For this review, use the dimensioned drawing (mm, ordinates from the lowest corner) and the shaded views. A direction names the side the tool comes from. Coordinates: 2 decimals unless noted, no trailing zeros. Order: outer loops, then holes, each group sorted by start corner. A loop starts at its lowest first (then second) coordinate and runs counter-clockwise, first axis right, second up. Notation, with made-up numbers: M -23,55 L 3,55 A19 ccw 3,74 Z; hole C 32,50.25 d2. An arc over 180 degrees is marked long. Answer in a Markdown table with one row per item.
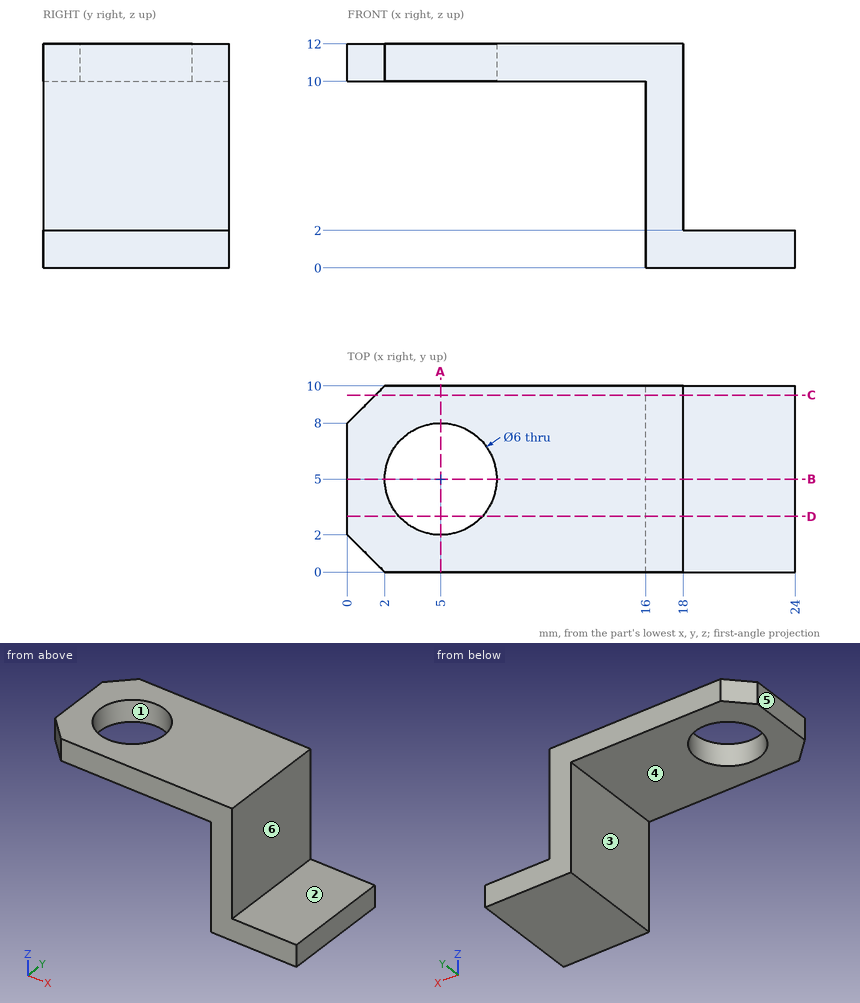
(1) Add section B-B, the plane y = 5. Give the boundary of the cut face in (x, z), and give its area (3 significant figures).
Return value:
| item | result |
|---|---|
| outline | M 0,10 L 2,10 L 2,12 L 0,12 Z; M 8,10 L 16,10 L 16,0 L 24,0 L 24,2 L 18,2 L 18,12 L 8,12 Z |
| area | 56.0 mm2 |
(2) Insertion check: pin 1 Ø5 at (y, z) = (4.5, 3) entering from -X; pin 2 Ø1.8 at (x, y) = (21, 4.5) entering from +Z; pin 3 Ø5 at (y, z) = (4, 7.5) entering from +X. Each pin has a flat end and moves straight along its axis. Give the tip position at first contact, or say it passes through.
Return value:
| item | result |
|---|---|
| pin 1 | stops at x = 16 |
| pin 2 | stops at z = 2 |
| pin 3 | stops at x = 18 |
(3) Add section D-D, the plane y = 3. Give the boundary of the cut face in (x, z).
Return value:
| item | result |
|---|---|
| outline | M 0,10 L 2.76,10 L 2.76,12 L 0,12 Z; M 7.24,10 L 16,10 L 16,0 L 24,0 L 24,2 L 18,2 L 18,12 L 7.24,12 Z |
(4) Draft analysis for pull direction X (two halves, no side actions). For the marked faces 1, 2 and 3, state which applies: pulls with the +X half, pulls with the -X half, needs draft (parallel to the pull), parting line crosses it, or undercut.
Return value:
| item | result |
|---|---|
| face 1 | undercut |
| face 2 | needs draft |
| face 3 | pulls with the -X half |
(5) Add section A-A, the plane x = 5. Give the boundary of the cut face in (y, z).
Return value:
| item | result |
|---|---|
| outline | M 0,10 L 2,10 L 2,12 L 0,12 Z; M 8,10 L 10,10 L 10,12 L 8,12 Z |
(6) Add section C-C, the plane y = 9.5. Give the boundary of the cut face in (x, z), and give its area (3 significant figures).
Return value:
| item | result |
|---|---|
| outline | M 1.5,10 L 16,10 L 16,0 L 24,0 L 24,2 L 18,2 L 18,12 L 1.5,12 Z |
| area | 65.0 mm2 |
(7) For the marked faces 4, 5 and 6, list the 3-axis set-ups (+Z, -Z, +X, -X, +Y, -Y) from which the entire face can be reached by the end or side of a thin tool; tool diameter is ignored.
Return value:
| item | result |
|---|---|
| face 4 | -Z, -X, +Y, -Y |
| face 5 | +Z, -Z, -X, +Y, -Y |
| face 6 | +Z, +X, +Y, -Y |
(8) For line 1 along Y through (x, z) = (5, 11.45); line 2 along X through (y, z) = (7.75, 6.5); line 3 along Z through (x, y) = (3.25, 7.5), list the stretches that pass through material, from the lowest coordinate up. Write a range as from..to.
Return value:
| item | result |
|---|---|
| line 1 | y = 0..2, 8..10 |
| line 2 | x = 16..18 |
| line 3 | z = 10..12 |
